```python
from build123d import *

# Parameters (mm, degrees)
EXTRUDE_1_DEPTH = 2


with BuildPart() as part:
    # Model → ﾎﾞｽ - 押し出し1 (new body)
    with BuildSketch(Plane.XY):
        Polygon((396.51989783, 60), (400, 60), (400, 61.22065558), (400, 140), (203.051638949, 199.084508315), (201, 199.7), (200, 200), (198.999999985, 199.699999996), (196.948361051, 199.084508315), (0, 140), (0, 61.22065558), (0, 60), (200, 60), align=None)
        Polygon((202.168514351, 197.261384393), (395.399063483, 62), (201, 62), (201, 197.611938698), align=None, mode=Mode.SUBTRACT)
        Polygon((2, 62.62065558), (2, 138.511938698), (191.728207796, 195.430401037), align=None, mode=Mode.SUBTRACT)
        Polygon((198.999999985, 197.611938694), (197.831485649, 197.261384393), (4.600936517, 62), (198.999999985, 62), align=None, mode=Mode.SUBTRACT)
        Polygon((398, 62.62065558), (398, 138.511938698), (208.271792204, 195.430401037), align=None, mode=Mode.SUBTRACT)
        Polygon((400, 0), (400, 58.955969334), (400, 60), (396.51989783, 60), (200, 60), (0, 60), (0, 58.955969334), (0, 0), align=None)
        Polygon((389.853231164, 58), (203.186564497, 2), (201, 2), (201, 58), align=None, mode=Mode.SUBTRACT)
        Polygon((210.146768888, 2), (396.813435555, 58), (398, 58), (398, 2), align=None, mode=Mode.SUBTRACT)
        Polygon((3.186564445, 58), (189.853231112, 2), (2, 2), (2, 58), align=None, mode=Mode.SUBTRACT)
        Polygon((196.813435503, 2), (198.999999985, 2), (198.999999985, 58), (10.146768836, 58), align=None, mode=Mode.SUBTRACT)
    extrude(amount=EXTRUDE_1_DEPTH)


solid = part.part
```
The listing builds one solid part. Answer for the finished solid, in the listing's coordinates (mm). Give positions to 0.01 mm unless a question says otherwise; leave off trailing zeros. Order: outer loops, then holes, each group sorted by start corner. A loop starts at its lowest first (then second) coordinate and runs counter-clockwise, first axis right, second up. Notation, with made-up numbers: (-10, 47) -> (20, 47) arc R6 cw to (20, 58) -> close; hole circle Ø9 at (36, -29.5). An arc over 180 degrees is marked (long way). Write each question's results on one line, items separated by ' | '.
Q1. The part is cut by section C-C, the plane x = 148.5. Give the vertices of the cut face in (y, z).
Checked values:
outline: (0, 0) -> (2, 0) -> (2, 2) -> (0, 2) -> close; (14.41, 0) -> (16.49, 0) -> (16.49, 2) -> (14.41, 2) -> close; (58, 0) -> (62, 0) -> (62, 2) -> (58, 2) -> close; (162.73, 0) -> (165.17, 0) -> (165.17, 2) -> (162.73, 2) -> close; (182.46, 0) -> (184.55, 0) -> (184.55, 2) -> (182.46, 2) -> close
Q2. Determine the mould class of faces 1 (the face through (102.6, 130.6, 1)), 2 (the face through (297.827, 30.392, 0.986)) for opening direction X: pulls with the +X half, pulls with the -X half, needs draft (parallel to the pull), parting line crosses it, or undercut.
Checked values:
face 1: undercut | face 2: undercut
Q3. The part is cut by section A-A, the plane y = 41.5. Give the vertices of the cut face in (x, z).
Checked values:
outline: (0, 0) -> (2, 0) -> (2, 2) -> (0, 2) -> close; (58.19, 0) -> (65.15, 0) -> (65.15, 2) -> (58.19, 2) -> close; (199, 0) -> (201, 0) -> (201, 2) -> (199, 2) -> close; (334.85, 0) -> (341.81, 0) -> (341.81, 2) -> (334.85, 2) -> close; (398, 0) -> (400, 0) -> (400, 2) -> (398, 2) -> close
Q4. Each of these flat-tipped pins is pushed along its axis until it touches: P1, Ø0.6, axis at x = 136.5, z = 1, coming from the -Y side; P2, Ø1, axis at x = 197.5, z = 1.5, coming from the +Y side; P3, Ø1, axis at x = 259, z = 1, coming from the +Y side; P4, Ø0.6, axis at x = 337, z = 1, coming from the +Y side. Where does it stop, or does it pass through?
Checked values:
P1: stops at y = 0 | P2: stops at y = 199.4 | P3: stops at y = 182.45 | P4: stops at y = 158.99
Q5. The part is cut by section B-B, the plane z = 0.5. State how many separate pieces and enclosed holes the cut face has, and give its area (3 significant figures).
Checked values:
separate pieces: 1 | enclosed holes: 8 | area: 5,860 mm^2
Q6. Straight lines are drawn through the part: probe 1 along X at (y, z) = (75, 1.65); probe 2 along Y at (x, z) = (245, 1.6); probe 3 along Y at (x, z) = (182, 1.8). For each, find the intervals that lie inside material, in ascending order. Write a range as from..to.
Checked values:
probe 1: x = 0..2, 19.68..23.17, 199..201, 376.83..380.32, 398..400 | probe 2: y = 0..2, 12.46..14.54, 58..62, 167.28..169.72, 184.41..186.5 | probe 3: y = 0..2, 4.36..6.44, 58..62, 186.18..188.62, 192.51..194.6
